from build123d import *

# Parameters (mm, degrees)
F0_R     = 4.75
F1_DEPTH = 4.5
F2_DEPTH = 1


# Not quite as in the source:
# - a feature names something its author has since deleted; it is built from what else it names


with BuildPart() as f1:
    # F0 (on Top) → F1 (new body)
    with BuildSketch(Plane.XY):
        with BuildLine():
            ThreePointArc((-15.8212677669, -17.7693802535), (0, -15.0870091218), (15.8212677669, -17.7693802535))
            ThreePointArc((15.8212677669, -17.7693802535), (44.9980398453, -0.2800041916), (16.3223672692, 18.019397609))
            ThreePointArc((16.3223672692, 18.019397609), (0, 15.1589625906), (-16.3223672692, 18.019397609))
            ThreePointArc((-16.3223672692, 18.019397609), (-44.9980398453, -0.2800041916), (-15.8212677669, -17.7693802535))
        make_face()
        with Locations((-27.7271234226, -12.8301069662)):
            Circle(F0_R, mode=Mode.SUBTRACT)
        with BuildLine():
            ThreePointArc((-11.8187225704, -10.0480051668), (-18.5761593137, -14.3529671553), (-19.6219637164, -6.409294062))
            ThreePointArc((-19.6219637164, -6.409294062), (-14.5612858272, -5.7430431784), (-11.8187225704, -10.0480051668))
        make_face(mode=Mode.SUBTRACT)
        with Locations((-36.7892470891, -5.75)):
            Circle(F0_R, mode=Mode.SUBTRACT)
        with Locations((16.5687225704, -10.0480051668)):
            Circle(F0_R, mode=Mode.SUBTRACT)
        with Locations((27.7271234226, -12.8301069662)):
            Circle(F0_R, mode=Mode.SUBTRACT)
        with Locations((36.7892470891, -5.75)):
            Circle(F0_R, mode=Mode.SUBTRACT)
        with BuildLine():
            ThreePointArc((-21.946758854, 3.6387111048), (-20.6950380116, 2.0074367433), (-20.25, 0))
            ThreePointArc((-20.25, 0), (-20.6950380116, -2.0074367433), (-21.946758854, -3.6387111048))
            ThreePointArc((-21.946758854, -3.6387111048), (-29.75, 0), (-21.946758854, 3.6387111048))
        make_face(mode=Mode.SUBTRACT)
        with Locations((-36.7892470891, 5.75)):
            Circle(F0_R, mode=Mode.SUBTRACT)
        with Locations((-27.7271234226, 12.8301069662)):
            Circle(F0_R, mode=Mode.SUBTRACT)
        with BuildLine():
            ThreePointArc((-11.8187225704, 10.0480051668), (-14.5612858272, 5.7430431784), (-19.6219637164, 6.409294062))
            ThreePointArc((-19.6219637164, 6.409294062), (-18.5761593137, 14.3529671553), (-11.8187225704, 10.0480051668))
        make_face(mode=Mode.SUBTRACT)
        with BuildLine():
            ThreePointArc((-11, 0), (0, 11), (11, 0))
            ThreePointArc((11, 0), (0, -11), (-11, 0))
        make_face(mode=Mode.SUBTRACT)
        with Locations((25, 0)):
            Circle(F0_R, mode=Mode.SUBTRACT)
        with Locations((36.7892470891, 5.75)):
            Circle(F0_R, mode=Mode.SUBTRACT)
        with Locations((16.5687225704, 10.0480051668)):
            Circle(F0_R, mode=Mode.SUBTRACT)
        with Locations((27.7271234226, 12.8301069662)):
            Circle(F0_R, mode=Mode.SUBTRACT)
    extrude(amount=F1_DEPTH)

    # F0 (on Top) → F2 (join)
    with BuildSketch(Plane.XY):
        with BuildLine():
            Line((-25, 0), (-20.25, 0))
            ThreePointArc((-20.25, 0), (-20.6950380116, 2.0074367433), (-21.946758854, 3.6387111048))
            Line((-21.946758854, 3.6387111048), (-25, 0))
        make_face()
        with BuildLine():
            Line((-25, 0), (-21.946758854, 3.6387111048))
            ThreePointArc((-21.946758854, 3.6387111048), (-29.75, 0), (-21.946758854, -3.6387111048))
            Line((-21.946758854, -3.6387111048), (-25, 0))
        make_face()
        with BuildLine():
            ThreePointArc((-21.946758854, -3.6387111048), (-20.6950380116, -2.0074367433), (-20.25, 0))
            Line((-20.25, 0), (-25, 0))
            Line((-25, 0), (-21.946758854, -3.6387111048))
        make_face()
        with Locations((25, 0)):
            Circle(F0_R)
        with BuildLine():
            ThreePointArc((-11.8187225704, 10.0480051668), (-18.5761593137, 14.3529671553), (-19.6219637164, 6.409294062))
            ThreePointArc((-19.6219637164, 6.409294062), (-14.5612858272, 5.7430431784), (-11.8187225704, 10.0480051668))
        make_face()
        with Locations((-27.7271234226, 12.8301069662)):
            Circle(F0_R)
        with Locations((-36.7892470891, 5.75)):
            Circle(F0_R)
        with Locations((-36.7892470891, -5.75)):
            Circle(F0_R)
        with Locations((-27.7271234226, -12.8301069662)):
            Circle(F0_R)
        with BuildLine():
            ThreePointArc((-11.8187225704, -10.0480051668), (-14.5612858272, -5.7430431784), (-19.6219637164, -6.409294062))
            ThreePointArc((-19.6219637164, -6.409294062), (-18.5761593137, -14.3529671553), (-11.8187225704, -10.0480051668))
        make_face()
        with Locations((16.5687225704, 10.0480051668)):
            Circle(F0_R)
        with Locations((27.7271234226, 12.8301069662)):
            Circle(F0_R)
        with Locations((36.7892470891, 5.75)):
            Circle(F0_R)
        with Locations((36.7892470891, -5.75)):
            Circle(F0_R)
        with Locations((27.7271234226, -12.8301069662)):
            Circle(F0_R)
        with Locations((16.5687225704, -10.0480051668)):
            Circle(F0_R)
    extrude(amount=F2_DEPTH)


solid = f1.part
Read the model definition and answer for the solid it produces. Units are mm, in the model's axes. A direction names the side the tool comes from. Round coordinates to 2 decimals unless told otherwise and drop trailing zeros. Write each loop counter-clockwise with the first axis right and the second up, starting at its lowest first coordinate (ties: lowest second). Pieces come first, ordered by that corner, then holes. Notation, with made-up numbers: (87.5, 52.5) - (101.5, 52.5) arc R20 ccw to (101.5, 70.5) - close; hole circle Ø3 at (82, 38.5). An arc over 180 degrees is marked (long way). Use a Markdown table: item, result.
(1) The part is cut by section B-B (x = -2.5). Write down the section's boundary in (y, z).
Reported:
| item | result |
|---|---|
| outline | (-15.15, 0) - (-10.71, 0) - (-10.71, 4.5) - (-15.15, 4.5) - close; (10.71, 0) - (15.22, 0) - (15.22, 4.5) - (10.71, 4.5) - close |
(2) Which of the six approach directions +Z, -Z, +X, -X, +Y, -Y give full straight-line access (tool end or side, diameter ignored) to faces 1 (the flat face through (-11, 5, 0)), 2 (the cylindrical face through (15.539, -14.685, 2.726))?
Reported:
| item | result |
|---|---|
| face 1 | -Z, +X, -X, +Y, -Y |
| face 2 | +Z |
(3) Straight lines are drawn through the part: line 1 along Y through (x, z) = (-17.5, 2.3); line 2 along Y through (x, z) = (-19, 3.05); line 3 along X through (y, z) = (-11.5, 1.55). For each, find the intervals that lie inside material, in ascending order. Write a range as [from, to].
Reported:
| item | result |
|---|---|
| line 1 | [-18.54, -14.71], [-5.39, 5.39], [14.71, 18.54] |
| line 2 | [-19.08, -14.13], [-5.97, 5.97], [14.13, 19.08] |
| line 3 | [-41.36, -32.29], [-23.17, -21.09], [-12.05, 12.05], [21.09, 23.17], [32.29, 41.36] |
(4) Each of these flat-tipped pins is pushed along its axis until it touches: pin 1 Ø1 at (x, z) = (15, 2) entering from +Y; pin 2 Ø7.5 at (x, y) = (-37.5, -6) entering from +Z; pin 3 Ø1.5 at (x, z) = (-6.5, 2.5) entering from +Y. Where does it stop, or does it pass through?
Reported:
| item | result |
|---|---|
| pin 1 | y = 17.73 |
| pin 2 | z = 1 |
| pin 3 | y = 15.71 |
(5) The mould has two halves that part along Y. Classify faces 3 (the flat face through (-11, -4, 4.5)), 4 (the flat face through (25, 0, 1)), 5 (the cylindrical face through (0.23, 15.16, 2.22)): released by +Y, released by -Y, zero draft, split by the parting line, or undercut.
Reported:
| item | result |
|---|---|
| face 3 | zero draft |
| face 4 | undercut |
| face 5 | released by +Y |
(6) The part is cut by section C-C (z = 3.7). State how many separate pieces and enclosed holes the cut face has, then the cut area to 3 significant figures.
Reported:
| item | result |
|---|---|
| separate pieces | 1 |
| enclosed holes | 15 |
| area | 1,600 mm2 |
(7) The part is cut by section A-A (y = 16). Write down the section's boundary in (x, z).
Reported:
| item | result |
|---|---|
| outline | (-37, 0) - (-8.95, 0) - (-8.95, 4.5) - (-24.19, 4.5) - (-24.19, 1) - (-31.26, 1) - (-31.26, 4.5) - (-37, 4.5) - close; (8.95, 0) - (37, 0) - (37, 4.5) - (31.26, 4.5) - (31.26, 1) - (24.19, 1) - (24.19, 4.5) - (8.95, 4.5) - close |
(8) The part is cut by section D-D (x = 25). Write down the section's boundary in (y, z).
Reported:
| item | result |
|---|---|
| outline | (-20, 0) - (20, 0) - (20, 4.5) - (16.72, 4.5) - (16.72, 1) - (8.94, 1) - (8.94, 4.5) - (4.75, 4.5) - (4.75, 1) - (-4.75, 1) - (-4.75, 4.5) - (-8.94, 4.5) - (-8.94, 1) - (-16.72, 1) - (-16.72, 4.5) - (-20, 4.5) - close |
